Here's how the part is built. I have some questions about the finished solid (model axes, mm). A direction names the side the tool comes from. Coordinates: 2 decimals unless noted, no trailing zeros. Write each loop counter-clockwise with the first axis right and the second up, starting at its lowest first coordinate (ties: lowest second). Pieces come first, ordered by that corner, then holes. Notation, with made-up numbers: (41.5, 29.5) -> (84.5, 29.5) arc R17 cw to (84.5, 42.5) -> close; hole circle Ø5 at (61, 60.5). An arc over 180 degrees is marked (long way). Put each result on its own line as item: value. Start each with the question number.
Item 1: On a 3-axis mill with a long thin cutter (end or side, diameter ignored), from which of +Z, -Z, +X, -X, +Y, -Y can I reach the whole of each face in a straight line? I mean faces 1 (the face through (-36, -8.238, 5)), 2 (the face through (-11, 11, 6)), 3 (the face through (12.282, 1, 5)), 4 (the face through (-12, -8.238, 8)), 5 (the face through (9.282, 0, 5)). Say none if no direction works.
Item 2: If we mould it in two halves opening along X, with no side actions, what happens to faces 6 (the face through (-37.718, 11, 5)), 7 (the face through (-11, -10, 6)), 8 (the face through (12, 1, 0))? For each: released by +X, released by -X, zero draft, split by the parting line, or undercut.
Item 3: For pin 1 (0.9 mm diameter, centred on x = -5.5, y = -10, fed in from -Z); pin 2 (5 mm diameter, centred on x = 8, z = 2, fed in from +Y); pin 3 (4 mm diameter, centred on y = 0.5, z = 5.5, fed in from +X); pin 4 (5 mm diameter, centred on y = -0.5, z = 6, fed in from -X), each with a flat end and sliding along its axis, tell me the tip position at first contact or that it passes through.
Item 4: I want a section at B-B, the plane z = 3.5. List the corners of the cut face in (x, y) for me.
Item 5: I want a section at A-A, the plane x = 3.5. List the corners of the cut face in (y, z) for me.
Item 6: I need wall thicknesses on line 1 (X direction, y = -3.5, z = 0.75); line 2 (Y direction, x = -20.5, z = 9). Which ranges of each line are inside material? Lowest first, please. Write a range as [from, to].
Item 7: I want a section at D-D, the plane z = 8.75. List the corners of the cut face in (x, y) for me, then the cut area to 3 significant figures.
Item 8: I want a section at C-C, the plane y = -5. List the corners of the cut face in (x, z) for me, then the cut area to 3 significant figures.
from build123d import *

# Parameters (mm, degrees)
SKETCH1_W           = 41
SKETCH1_H           = 17.79
BOSS_EXTRUDE1_DEPTH = 10
SKETCH10_W          = 41
SKETCH10_H          = 3
CUT_EXTRUDE1_DEPTH  = 6


with BuildPart() as part:
    # Sketch1 → Boss-Extrude1 (new body)
    with BuildSketch(Plane.XY):
        Polygon((12.281684518, 9.551958914), (15.281684518, 9.551958914), (15.281684518, 12.551958914), (-37.718315482, 12.551958914), (-37.718315482, 9.551958914), (-34.718315482, 9.551958914), (-34.718315482, -8.238041086), (-37.718315482, -8.238041086), (-37.718315482, -11.238041086), (15.281684518, -11.238041086), (15.281684518, -8.238041086), (12.281684518, -8.238041086), align=None)
        with Locations((-11.218315482, 0.656958914)):
            Rectangle(SKETCH1_W, SKETCH1_H, mode=Mode.SUBTRACT)
    extrude(amount=BOSS_EXTRUDE1_DEPTH)

    # Sketch10 → Cut-Extrude1 (cut)
    with BuildSketch(Plane(origin=(0, 0, 0), x_dir=(-1, 0, 0), z_dir=(0, 0, -1))):
        with Locations((11.218315482, -9.738041086)):
            Rectangle(SKETCH10_W, SKETCH10_H)
    cut_extrude1 = extrude(amount=-CUT_EXTRUDE1_DEPTH, mode=Mode.SUBTRACT)

    # Mirror3: Cut-Extrude1 across plane
    add(cut_extrude1.mirror(Plane.ZX.offset(0.656958914)), mode=Mode.SUBTRACT)


solid = part.part
Calculated:
1. face 1: +Z, -Z, -X
1. face 2: -Z, +Y, -Y
1. face 3: +Z, -Z, +X
1. face 4: +Z, -Z
1. face 5: -Z
2. face 6: released by -X
2. face 7: undercut
2. face 8: zero draft
3. pin 1: stops at z = 6
3. pin 2: stops at y = 12.55
3. pin 3: stops at x = 12.28
3. pin 4: stops at x = -34.72
4. outline: (-37.72, -11.24) -> (-31.72, -11.24) -> (-31.72, 12.55) -> (-37.72, 12.55) -> (-37.72, 9.55) -> (-34.72, 9.55) -> (-34.72, -8.24) -> (-37.72, -8.24) -> close; (9.28, -11.24) -> (15.28, -11.24) -> (15.28, -8.24) -> (12.28, -8.24) -> (12.28, 9.55) -> (15.28, 9.55) -> (15.28, 12.55) -> (9.28, 12.55) -> close
5. outline: (-11.24, 6) -> (-8.24, 6) -> (-8.24, 10) -> (-11.24, 10) -> close; (9.55, 6) -> (12.55, 6) -> (12.55, 10) -> (9.55, 10) -> close
6. line 1: x = [-34.72, -31.72], [9.28, 12.28]
6. line 2: y = [-11.24, -8.24], [9.55, 12.55]
7. outline: (-37.72, -11.24) -> (15.28, -11.24) -> (15.28, -8.24) -> (12.28, -8.24) -> (12.28, 9.55) -> (15.28, 9.55) -> (15.28, 12.55) -> (-37.72, 12.55) -> (-37.72, 9.55) -> (-34.72, 9.55) -> (-34.72, -8.24) -> (-37.72, -8.24) -> close; hole (-31.72, -8.24) -> (9.28, -8.24) -> (9.28, 9.55) -> (-31.72, 9.55) -> close
7. area: 425 mm2
8. outline: (-34.72, 0) -> (-31.72, 0) -> (-31.72, 10) -> (-34.72, 10) -> close; (9.28, 0) -> (12.28, 0) -> (12.28, 10) -> (9.28, 10) -> close
8. area: 60.0 mm2
